```python
from build123d import *

# Parameters (mm, degrees)
SZKIC1_W                       = 47
SZKIC1_H                       = 39.6
DODANIE_WYCI_GNI_CIE3_DEPTH    = 75
SZKIC4_R                       = 8.15
DODANIE_WYCI_GNI_CIE4_DEPTH    = 10
SZKIC5_R                       = 8.15
DODANIE_WYCI_GNI_CIE5_DEPTH    = 5
OTW_R_GWINTOWANY_M4X0_71_D     = 3.3
OTW_R_GWINTOWANY_M4X0_71_DEPTH = 15
OTW_R_GWINTOWANY_M4X0_71_TIP   = 0.991420021
SFAZOWANIE1_SIZE               = 0.5


with BuildPart() as part:
    # Szkic1 → Dodanie-wyciągnięcie3 (new body)
    with BuildSketch(Plane.XY):
        with Locations((23.5, 19.8)):
            Rectangle(SZKIC1_W, SZKIC1_H)
    extrude(amount=DODANIE_WYCI_GNI_CIE3_DEPTH)

    # Szkic4 → Dodanie-wyciągnięcie4 (add)
    with BuildSketch(Plane(origin=(0, 0, 27.5), x_dir=(-1, 0, 0), z_dir=(0, 0, -1))):
        with BuildLine():
            Line((-47, 39.6), (-68.5, 39.6))
            ThreePointArc((-68.5, 39.6), (-88.3, 19.8), (-68.5, 0))
            Line((-68.5, 0), (-47, 0))
            Line((-47, 0), (-47, 39.6))
        make_face()
        with Locations((-68.5, 19.8)):
            Circle(SZKIC4_R, mode=Mode.SUBTRACT)
        with BuildLine():
            Line((21.5, 0), (0, 0))
            Line((0, 0), (0, 39.6))
            Line((0, 39.6), (21.5, 39.6))
            ThreePointArc((21.5, 39.6), (41.3, 19.8), (21.5, 0))
        make_face()
        with Locations((21.5, 19.8)):
            Circle(SZKIC4_R, mode=Mode.SUBTRACT)
    dodanie_wyci_gni_cie4 = extrude(amount=DODANIE_WYCI_GNI_CIE4_DEPTH)

    # Lustro1: Dodanie-wyciągnięcie4 across plane
    add(dodanie_wyci_gni_cie4.mirror(Plane(origin=(0, 0, 37.5), x_dir=(1, 0, 0), z_dir=(0, 0, -1))))

    # Szkic5 → Dodanie-wyciągnięcie5 (add)
    with BuildSketch(Plane(origin=(0, 0, 22.5), x_dir=(-1, 0, 0), z_dir=(0, 0, -1))):
        with BuildLine():
            Line((-47, 0), (0, 0))
            Line((0, 0), (0, -20))
            ThreePointArc((0, -20), (-23.5, -43.5), (-47, -20))
            Line((-47, -20), (-47, 0))
        make_face()
        with Locations((-23.5, -20)):
            Circle(SZKIC5_R, mode=Mode.SUBTRACT)
    dodanie_wyci_gni_cie5 = extrude(amount=DODANIE_WYCI_GNI_CIE5_DEPTH)

    # Lustro2: Dodanie-wyciągnięcie5 across plane
    add(dodanie_wyci_gni_cie5.mirror(Plane(origin=(0, 0, 37.5), x_dir=(1, 0, 0), z_dir=(0, 0, -1))))

    # Otwór gwintowany M4x0.71
    with Locations(Plane.XY.offset(75)):
        with Locations((4.5, 34.8), (23.5, 32.8), (42.5, 34.8), (42.5, 4.8), (23.5, 6.8), (4.5, 4.8)):
            Hole(OTW_R_GWINTOWANY_M4X0_71_D / 2, depth=OTW_R_GWINTOWANY_M4X0_71_DEPTH)
            with Locations((0, 0, -(OTW_R_GWINTOWANY_M4X0_71_DEPTH + OTW_R_GWINTOWANY_M4X0_71_TIP / 2))):  # 118° drill point
                Cone(0, OTW_R_GWINTOWANY_M4X0_71_D / 2, OTW_R_GWINTOWANY_M4X0_71_TIP, mode=Mode.SUBTRACT)

    # Sfazowanie1
    sfazowanie1_edges = [part.edges().sort_by_distance(p)[0] for p in [
        (6.15, 4.8, 75),
        (25.15, 6.8, 75),
        (44.15, 4.8, 75),
        (44.15, 34.8, 75),
        (25.15, 32.8, 75),
        (6.15, 34.8, 75),
    ]]
    chamfer(sfazowanie1_edges, length=SFAZOWANIE1_SIZE)


solid = part.part
```
Source: CAD feature listing. Evaluate the final solid. Frame: model axes, mm. A direction names the side the tool comes from. Round coordinates to 2 decimals unless told otherwise and drop trailing zeros. Loops run counter-clockwise (first coordinate to the right, second up) from the corner with the lowest first, then second, coordinate; pieces in that order, holes last.
1. Section query D-D on x = 71. Output: boundary loops of the cut face in (y, z), and give its area (3 significant figures).
2. Section query C-C on y = -37. Output: boundary loops of the cut face in (x, z).
3. Section query B-B on x = 53. Output: boundary loops of the cut face in (y, z), and give its area (3 significant figures).
4. Contact query for flat-ended pins moving along their axis: pin 1 (5 mm diameter, centred on y = -1.5, z = 11, fed in from -X); pin 2 (6 mm diameter, centred on x = 46, z = 63.5, fed in from -Y); pin 3 (4.5 mm diameter, centred on x = 42.5, y = 4.8, fed in from -Z); pin 4 (10 mm diameter, centred on y = 27, z = 39.5, fed in from +X). Output: stop coordinate, or through.
5. Ray query, L1, parallel to X at y = 4.8, z = 69.5; L2, parallel to Y at x = 42.5, z = 65; L3, parallel to Z at x = 56, y = 34. Return the intervals inside material, ascending.
6. Access query for faces 4 (the flat face through (-12, 20, 27.5)), 5 (the flat face through (17.9, -26.3, 52.5)), 6 (the flat face through (0, -10, 20)), 7 (the flat face through (47, 20, 66)). Directions: +Z, -Z, +X, -X, +Y, -Y. A direction counts if a zero-diameter tool reaches every point of the face in a straight line with its end or side. Return the directions, or none.
7. Mould query, pull axis Z, two halves, no side actions, for faces 1 (the flat face through (-12, 20, 47.5)), 2 (the conical face through (42.29, 34.99, 59.18)), 3 (the cylindrical face through (44.15, 34.87, 67.15)). Classes: released by +Z, released by -Z, zero draft, split by the parting line, or undercut.
8. Section query A-A on z = 67. Output: boundary loops of the cut face in (x, y).
Answers below:
1. outline: (0.16, 17.5) - (12.04, 17.5) - (12.04, 27.5) - (0.16, 27.5) - close; (0.16, 47.5) - (12.04, 47.5) - (12.04, 57.5) - (0.16, 57.5) - close; (27.56, 17.5) - (39.44, 17.5) - (39.44, 27.5) - (27.56, 27.5) - close; (27.56, 47.5) - (39.44, 47.5) - (39.44, 57.5) - (27.56, 57.5) - close
1. area: 475 mm2
2. outline: (7.28, 17.5) - (39.72, 17.5) - (39.72, 22.5) - (7.28, 22.5) - close; (7.28, 52.5) - (39.72, 52.5) - (39.72, 57.5) - (7.28, 57.5) - close
3. outline: (0, 17.5) - (39.6, 17.5) - (39.6, 27.5) - (0, 27.5) - close; (0, 47.5) - (39.6, 47.5) - (39.6, 57.5) - (0, 57.5) - close
3. area: 792 mm2
4. pin 1: stops at x = 0
4. pin 2: stops at y = 0
4. pin 3: stops at z = 0
4. pin 4: stops at x = 47
5. L1: x = 0 to 2.85, 6.15 to 40.85, 44.15 to 47
5. L2: y = 0 to 3.15, 6.45 to 33.15, 36.45 to 39.6
5. L3: z = 17.5 to 27.5, 47.5 to 57.5
6. face 4: -X, +Y, -Y
6. face 5: +X, -X, -Y
6. face 6: +Z, -Z, -X, -Y
6. face 7: +Z, +X, +Y, -Y
7. face 1: undercut
7. face 2: released by +Z
7. face 3: zero draft
8. outline: (0, 0) - (47, 0) - (47, 39.6) - (0, 39.6) - close; hole circle Ø3.3 at (4.5, 4.8); hole circle Ø3.3 at (4.5, 34.8); hole circle Ø3.3 at (23.5, 6.8); hole circle Ø3.3 at (23.5, 32.8); hole circle Ø3.3 at (42.5, 4.8); hole circle Ø3.3 at (42.5, 34.8)
